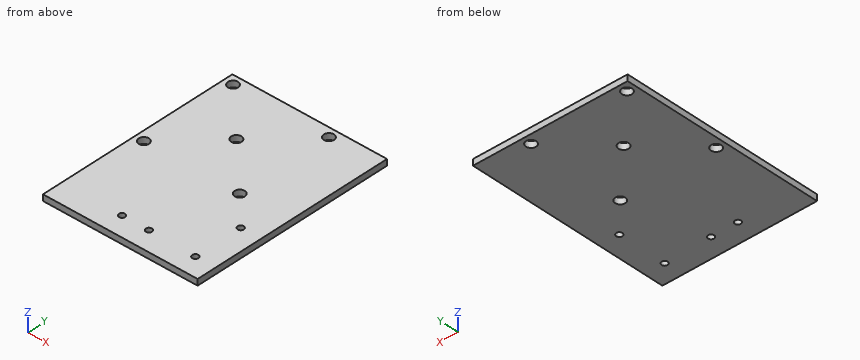
```python
from build123d import *

# Parameters (mm, degrees)
SKETCH1_W           = 75.9
SKETCH1_H           = 100
BOSS_EXTRUDE1_DEPTH = 3
SKETCH2_R           = 2.5
CUT_EXTRUDE1_DEPTH  = 10
SKETCH5_R           = 1.5
CUT_EXTRUDE2_DEPTH  = 10
SKETCH7_R           = 1.5
CUT_EXTRUDE3_DEPTH  = 19.8
SKETCH8_R           = 2.5
CUT_EXTRUDE4_DEPTH  = 10


with BuildPart() as part:
    # Sketch1 → Boss-Extrude1 (new body)
    with BuildSketch(Plane.XY):
        with Locations((37.95, 50)):
            Rectangle(SKETCH1_W, SKETCH1_H)
    extrude(amount=BOSS_EXTRUDE1_DEPTH)

    # Sketch2 → Cut-Extrude1 (cut)
    with BuildSketch(Plane(origin=(0, 0, 0), x_dir=(-1, 0, 0), z_dir=(0, 0, -1))):
        with Locations((-51.538582233, 95.538582233)):
            Circle(SKETCH2_R)
        with Locations((-4.461417767, 95.538582233)):
            Circle(SKETCH2_R)
        with Locations((-4.461417767, 48.461417767)):
            Circle(SKETCH2_R)
        with Locations((-51.538582233, 48.461417767)):
            Circle(SKETCH2_R)
    extrude(amount=-CUT_EXTRUDE1_DEPTH, mode=Mode.SUBTRACT)

    # Sketch5 → Cut-Extrude2 (cut)
    with BuildSketch(Plane.XY.offset(3)):
        with Locations((66, 33.391370051)):
            Circle(SKETCH5_R)
        with Locations((66, 9.470993714)):
            Circle(SKETCH5_R)
    extrude(amount=-CUT_EXTRUDE2_DEPTH, mode=Mode.SUBTRACT)

    # Sketch7 → Cut-Extrude3 (cut)
    with BuildSketch(Plane(origin=(0, 0, 0), x_dir=(-1, 0, 0), z_dir=(0, 0, -1))):
        with Locations((-29.6, 9.9)):
            Circle(SKETCH7_R)
        with Locations((-42.8, 9.9)):
            Circle(SKETCH7_R)
    extrude(amount=-CUT_EXTRUDE3_DEPTH, mode=Mode.SUBTRACT)

    # Sketch8 → Cut-Extrude4 (cut)
    with BuildSketch(Plane(origin=(0, 0, 0), x_dir=(-1, 0, 0), z_dir=(0, 0, -1))):
        with Locations((-28, 72)):
            Circle(SKETCH8_R)
    extrude(amount=-CUT_EXTRUDE4_DEPTH, mode=Mode.SUBTRACT)


solid = part.part
```
Source: CAD feature listing. Evaluate the final solid. Frame: model axes, mm. Give positions to 0.01 mm unless a question says otherwise; leave off trailing zeros. Order: outer loops, then holes, each group sorted by start corner. A loop starts at its lowest first (then second) coordinate and runs counter-clockwise, first axis right, second up.
(1) Contact query for a flat-ended pin moving along its axis: P1, Ø3, axis at x = 4.46, y = 95.54, coming from the +Z side. Output: stop coordinate, or through.
(2) Section query D-D (z = 1.8). State how many separate pieces and enclosed holes the cut face has, plus the area to 3 significant figures.
(3) Section query A-A (y = 72). Return the cut outline in (x, z).
(4) Section query B-B (x = 42.8). Return the cut outline in (y, z), plus the area to 3 significant figures.
(5) Material intervals for line 1 along Y through (x, z) = (6.5, 1.45); line 2 along Y through (x, z) = (28, 2.35); line 3 along Y through (x, z) = (29.5, 1.2), sorted ascending.
(6) Section query C-C (x = 66). Return the cut outline in (y, z).
Outcome:
1. P1: passes through
2. separate pieces: 1
2. enclosed holes: 9
2. area: 7,460 mm2
3. outline: (0, 0) - (25.5, 0) - (25.5, 3) - (0, 3) - close; (30.5, 0) - (75.9, 0) - (75.9, 3) - (30.5, 3) - close
4. outline: (0, 0) - (8.4, 0) - (8.4, 3) - (0, 3) - close; (11.4, 0) - (100, 0) - (100, 3) - (11.4, 3) - close
4. area: 291 mm2
5. line 1: y = 0 to 47.01, 49.91 to 94.09, 96.99 to 100
5. line 2: y = 0 to 69.5, 74.5 to 100
5. line 3: y = 0 to 8.4, 11.4 to 70, 74 to 100
6. outline: (0, 0) - (7.97, 0) - (7.97, 3) - (0, 3) - close; (10.97, 0) - (31.89, 0) - (31.89, 3) - (10.97, 3) - close; (34.89, 0) - (100, 0) - (100, 3) - (34.89, 3) - close
